For this review, take the finished solid that the model builds, in its own axes (mm). Face numbers are marked on the shaded views. A direction names the side the tool comes from. Coordinates: 2 decimals unless noted, no trailing zeros. Loops run counter-clockwise (first coordinate to the right, second up) from the corner with the lowest first, then second, coordinate; pieces in that order, holes last. Notation, with made-up numbers: (5.25, 23) -> (29.25, 23) arc R13 ccw to (29.25, 42) -> close; hole circle Ø8 at (76.5, 38). An arc over 180 degrees is marked (long way). One line per item, written item: value.
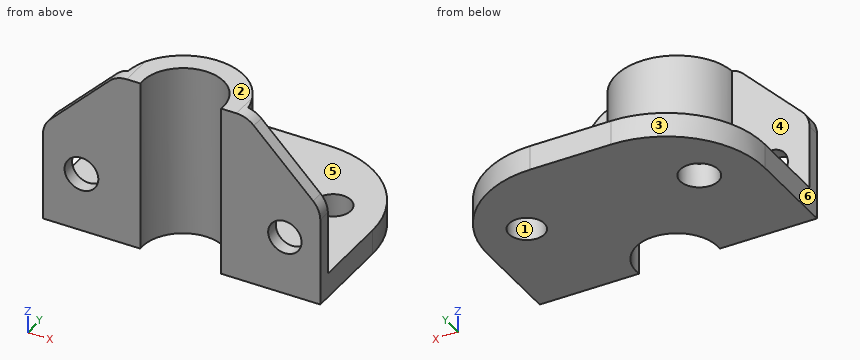
Autodesk Inventor part; units mm, degrees
ref_plane "YZ Plane" through (0, 0, 0) normal (1, 0, 0) x (0, 1, 0)
ref_plane "XZ Plane" through (0, 0, 0) normal (0, 1, 0) x (-1, 0, 0)
ref_plane "XY Plane" through (0, 0, 0) normal (0, 0, 1) x (1, 0, 0)
sketch "스케치1" plane through (0, 0, 0) normal (0, 0, 1) x (1, 0, 0)
  line L0 (28.2247, -19.3821) -> (-28.2247, -19.3821)
  line L1 (-28.2247, -19.3821) -> (-28.2247, 19.3821)
  line L2 (-28.2247, 19.3821) -> (28.2247, 19.3821)
  line L3 (28.2247, 19.3821) -> (28.2247, -19.3821)
  line L4 (28.2247, -19.3821) -> (-28.2247, 19.3821) construction
  line L5 (-28.2247, -19.3821) -> (28.2247, 19.3821) construction
  point P0 (0, 0)
extrude "돌출1" add sketch "스케치1" along normal blind 35
sketch "스케치2" plane through (0, 0, 35) normal (0, 0, 1) x (1, 0, 0)
  line L0 (-28.2247, -19.3821) -> (28.2247, -19.3821)
  arc A0 (8.0086, -19.3821) -> (-8.4193, -19.3821) centre (-0.2053, -18.5165) ccw
  arc A1 (12.0005, -16.6695) -> (-12.4112, -16.6695) centre (-0.2053, -18.5165) ccw
  line L1 (28.2247, -19.3821) -> (28.2247, 19.3821)
  line L2 (28.2247, -16.6695) -> (12.0005, -16.6695)
  line L3 (-12.4112, -16.6695) -> (-28.2247, -16.6695)
  line L4 (28.2247, -16.6695) -> (28.2247, 19.3821)
  line L5 (28.2247, 19.3821) -> (-28.2247, 19.3821)
  line L6 (-28.2247, 19.3821) -> (-28.2247, -16.6695)
  point P0 (0, 0)
extrude "돌출2" cut sketch "스케치2" against normal blind 30 contours L2 A1 L3 L6 L5 L1
extrude "돌출3" cut sketch "스케치2" against normal blind 35 contours A0 L0
sketch "스케치3" plane through (-28.2247, -16.6695, 35) normal (0, 1, 0) x (1, 0, 0)
  circle A0 centre (7.8268, 23.0556) radius 3.4368
  circle A1 centre (49.2387, 23.0556) radius 3.3984
  point P0 (28.2247, 35)
extrude "돌출4" cut sketch "스케치3" against normal blind 35
chamfer "모따기1" distance 15 angle 45 1 edges at (-28.2247, -18.0258, 35)
chamfer "모따기2" distance 15 angle 45 1 edges at (28.2247, -18.0258, 35)
fillet "모깎기1" radius 5 4 edges at (28.2247, -18.0258, 20) (13.2247, -18.0258, 35) (-13.2247, -18.0258, 35) (-28.2247, -18.0258, 20)
sketch "스케치4" plane through (0, 0, 5) normal (0, 0, 1) x (1, 0, 0)
  circle A0 centre (18.185, 3.0025) radius 3.5989
  circle A1 centre (-16.9318, 3.0025) radius 3.8942
  line L0 (-28.2247, 19.3821) -> (28.2247, 19.3821)
  arc A2 (-10.8118, 19.3821) -> (-28.2247, -16.6695) centre (16.7776, -16.1746) ccw
  line L1 (28.2247, 19.3821) -> (28.2247, -19.3821)
  arc A3 (28.2247, -16.6695) -> (8.7119, 19.3821) centre (-7.9765, -12.9568) ccw
  line L2 (-28.2247, -16.6695) -> (-28.2247, 19.3821)
  line L3 (-28.2247, -16.6695) -> (-28.2247, 19.3821)
  line L4 (-28.2247, 19.3821) -> (-10.8118, 19.3821)
  line L5 (8.7119, 19.3821) -> (28.2247, 19.3821)
  point P0 (0, 0)
extrude "돌출5" cut sketch "스케치4" against normal blind 35 contours A0 | A1
sketch "스케치5" plane through (0, 0, 0) normal (0, 0, -1) x (-1, 0, 0)
  point P0 (0, 0)
fillet "모깎기2" radius 20 2 edges at (28.2247, 19.3821, 2.5) (-28.2247, 19.3821, 2.5)
properties part number "240516_3Dsketch02"
1. For the marked faces 4, 5 and 6, list the 3-axis set-ups (+Z, -Z, +X, -X, +Y, -Y) from which the entire face can be reached by the end or side of a thin tool; tool diameter is ignored.
Return value:
face 4: +Z, -X, +Y
face 5: +Z, +Y
face 6: +Z, -Z, -X, +Y, -Y
2. The part is to be moulded in two halves that separate along X. For the marked faces 1, 2 and 3, say which applies: pulls with the +X half, pulls with the -X half, needs draft (parallel to the pull), parting line crosses it, or undercut.
Return value:
face 1: undercut
face 2: needs draft
face 3: pulls with the -X half
3. Take a section at C-C, the plane x = 23. Give the boundary of the cut face in (y, z), and give its area (3 significant figures).
Return value:
outline: (-19.38, 0) -> (12.86, 0) -> (12.86, 5) -> (-16.67, 5) -> (-16.67, 9.19) -> (-19.38, 9.19) -> close; (-19.38, 14.7) -> (-16.67, 14.7) -> (-16.67, 25.22) -> (-19.38, 25.22) -> close
area: 201 mm2
4. Take a section at D-D, the plane z = 13. Give the boundary of the cut face in (x, y), and give its area (3 significant figures).
Return value:
outline: (-28.22, -19.38) -> (-23.67, -19.38) -> (-23.67, -16.67) -> (-28.22, -16.67) -> close; (-17.13, -19.38) -> (-8.42, -19.38) arc R8.26 cw (long way) to (8.01, -19.38) -> (17.78, -19.38) -> (17.78, -16.67) -> (12, -16.67) arc R12.34 ccw to (-12.41, -16.67) -> (-17.13, -16.67) -> close; (24.24, -19.38) -> (28.22, -19.38) -> (28.22, -16.67) -> (24.24, -16.67) -> close
area: 190 mm2
5. Insertion check: pin 1 Ø1 at (y, z) = (-15, 6) entering from -X; pin 2 Ø1 at (x, y) = (-18.5, 6.5) entering from +Z; pin 3 Ø4 at (y, z) = (3.5, 3.5) entering from -X. Each pin has a flat end and moves straight along its axis. Give the tip position at first contact, or say it passes through.
Return value:
pin 1: stops at x = -12.18
pin 2: stops at z = 5
pin 3: stops at x = -28.11
6. Take a section at A-A, the plane z = 4. Give the boundary of the cut face in (x, y) (1 decimal).
Return value:
outline: (-28.2, -19.4) -> (-8.4, -19.4) arc R8.3 cw (long way) to (8, -19.4) -> (28.2, -19.4) -> (28.2, -0.6) arc R20 ccw to (8.2, 19.4) -> (-8.2, 19.4) arc R20 ccw to (-28.2, -0.6) -> close; hole circle Ø7.8 at (-16.9, 3); hole circle Ø7.2 at (18.2, 3)
7. To check wall thickness, follow probe 1 along Y at (x, z) = (24.5, 12); probe 2 along Z at (x, y) = (-22.5, 1); probe 3 along X at (y, z) = (-16, 32). State the ranges of each line that lie inside material, in increasing order. Write a range as from..to.
Return value:
probe 1: y = -19.38..-16.67
probe 2: z = 0..5
probe 3: x = -12.29..-8.07, 7.66..11.88
8. Take a section at B-B, the plane y = 1. Give the boundary of the cut face in (x, z).
Return value:
outline: (-28.16, 0) -> (-20.27, 0) -> (-20.27, 5) -> (-28.16, 5) -> close; (-13.59, 0) -> (15.19, 0) -> (15.19, 5) -> (-13.59, 5) -> close; (21.18, 0) -> (28.16, 0) -> (28.16, 5) -> (21.18, 5) -> close
